from build123d import *

# Parameters (mm, degrees)
SKETCH_1_W             = 248
SKETCH_1_H             = 80
SM_BASE_FLANGE_1_DEPTH = 3
SKETCH_6_R             = 2
CUT_EXTRUDE_1_DEPTH    = 10
OTHER_START            = -40
OTHER_1_DEPTH          = 80
OTHER_1_2_DEPTH        = 80
CUT_EXTRUDE_2_DEPTH    = 10
FILLET_1_R             = 5


# Read off the part's stored shape, not the designer's step: 绘制的折弯1
# Sheet-metal steps are written as plain solids
with BuildPart() as part:
    # Sketch 1 → 基体-法兰1 (new body)
    with BuildSketch(Plane.XY):
        Rectangle(SKETCH_1_W, SKETCH_1_H)
    extrude(amount=-SM_BASE_FLANGE_1_DEPTH)

    # 草图6 → 切除-拉伸1 (cut)
    with BuildSketch(Plane.XY):
        with Locations((-97, 32)):
            Circle(SKETCH_6_R)
        with Locations((-76, 31)):
            Circle(SKETCH_6_R)
        with Locations((97, 32)):
            Circle(SKETCH_6_R)
        with Locations((76, 31)):
            Circle(SKETCH_6_R)
        with Locations((76, -31)):
            Circle(SKETCH_6_R)
        with Locations((97, -32)):
            Circle(SKETCH_6_R)
        with Locations((-97, -32)):
            Circle(SKETCH_6_R)
        with Locations((-76, -31)):
            Circle(SKETCH_6_R)
    extrude(amount=-CUT_EXTRUDE_1_DEPTH, mode=Mode.SUBTRACT)

    # Other 1 outline → Other 1 (cut)
    with BuildSketch(Plane(origin=(0, 0, 0), x_dir=(1, 0, 0), z_dir=(0, 1, 0)).offset(OTHER_START)):
        with BuildLine():
            Line((124, 3), (109, 3))
            ThreePointArc((109, 3), (112, 2.196152423), (114.196152423, 0))
            Line((114.196152423, 0), (124, 0))
            Line((124, 0), (124, 3))
        make_face()
        with BuildLine():
            ThreePointArc((-114.196152423, 0), (-112, 2.196152423), (-109, 3))
            Line((-109, 3), (-124, 3))
            Line((-124, 3), (-124, 0))
            Line((-124, 0), (-114.196152423, 0))
        make_face()
    extrude(amount=OTHER_1_DEPTH, mode=Mode.SUBTRACT)

    # Other 1 2 outline → Other 1 2 (add)
    with BuildSketch(Plane(origin=(0, 0, 0), x_dir=(1, 0, 0), z_dir=(0, 1, 0)).offset(OTHER_START)):
        with BuildLine():
            ThreePointArc((115, -3), (114.795554958, -1.447085729), (114.196152423, 0))
            Line((114.196152423, 0), (109, 0))
            ThreePointArc((109, 0), (111.121320344, -0.878679656), (112, -3))
            Line((112, -3), (112, -10.931416529))
            Line((112, -10.931416529), (115, -10.931416529))
            Line((115, -10.931416529), (115, -3))
        make_face()
        with BuildLine():
            Line((-109, 0), (-114.196152423, 0))
            ThreePointArc((-114.196152423, 0), (-114.795554958, -1.447085729), (-115, -3))
            Line((-115, -3), (-115, -10.931416529))
            Line((-115, -10.931416529), (-112, -10.931416529))
            Line((-112, -10.931416529), (-112, -3))
            ThreePointArc((-112, -3), (-111.121320344, -0.878679656), (-109, 0))
        make_face()
    extrude(amount=OTHER_1_2_DEPTH)

    # 草图8 → 切除-拉伸2 (cut)
    with BuildSketch(Plane(origin=(0, 0, -3), x_dir=(-1, 0, 0), z_dir=(0, 0, -1))):
        with BuildLine():
            Line((-52, 25), (52, 25))
            ThreePointArc((52, 25), (77, 0), (52, -25))
            Line((52, -25), (-52, -25))
            ThreePointArc((-52, -25), (-77, 0), (-52, 25))
        make_face()
    extrude(amount=-CUT_EXTRUDE_2_DEPTH, mode=Mode.SUBTRACT)

    # 圆角1
    fillet_1_edges = [part.edges().sort_by_distance(p)[0] for p in [
        (113.5, 40, 10.931416529),
        (113.5, -40, 10.931416529),
        (-113.5, -40, 10.931416529),
        (-113.5, 40, 10.931416529),
    ]]
    fillet(fillet_1_edges, radius=FILLET_1_R)


solid = part.part
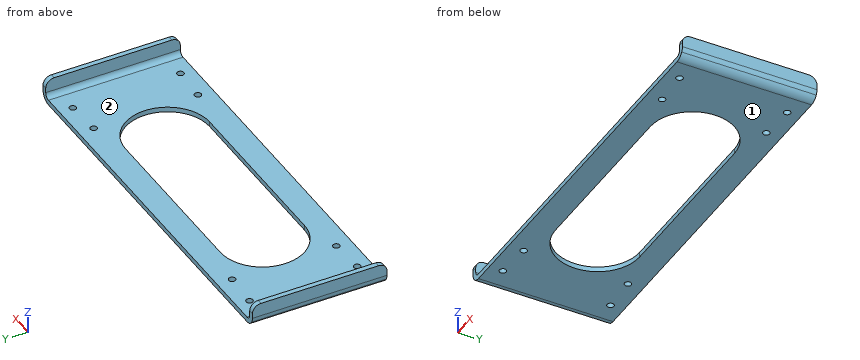
Could you check a few things on this model? Use its own coordinates, in mm. Face numbers are marked on the shaded views. Give positions to 0.01 mm unless a question says otherwise; leave off trailing zeros. Order: outer loops, then holes, each group sorted by start corner. A loop starts at its lowest first (then second) coordinate and runs counter-clockwise, first axis right, second up. Notation, with made-up numbers: (-1, 29) -> (27, 29) arc R26 cw to (27, 54) -> close; hole circle Ø2 at (65, 11.5). An arc over 180 degrees is marked (long way). Answer in a Markdown table with one row per item. Add a question column.
Item 1: Imagine slicing it at C-C (x = 97). List the corners of the cut face in (y, z) for me, and give its area (3 significant figures).
Item 2: Imagine slicing it at D-D (y = -19). List the corners of the cut face in (x, z) for me.
Item 3: We'd pull the mould along X, two halves only. Please class the marked faces 1 and 2: pulls with the +X half, pulls with the -X half, needs draft (parallel to the pull), parting line crosses it, or undercut.
Item 4: Imagine slicing it at A-A (y = 0). List the corners of the cut face in (x, z) for me.
Item 5: Imagine slicing it at B-B (x = 12.5). List the corners of the cut face in (y, z) for me, and give its area (3 significant figures).
Item 6: Please list where these lines run through material, in increasing order: probe 1 along Y at (x, z) = (97, -0.8); probe 2 along X at (y, z) = (3, 9); probe 3 along Y at (x, z) = (48, -1).
Item 7: I'm going to push a flat-ended pin straight in: P1, Ø4.5, axis at x = 76, y = -31, coming from the +Z side. Where does the tip first touch, or does it pass through?
Result:
| question | item | result |
|---|---|---|
| 1 | outline | (-40, -3) -> (-34, -3) -> (-34, 0) -> (-40, 0) -> close; (-30, -3) -> (30, -3) -> (30, 0) -> (-30, 0) -> close; (34, -3) -> (40, -3) -> (40, 0) -> (34, 0) -> close |
| 1 | area | 216 mm2 |
| 2 | outline | (-115, 3) arc R6 ccw to (-109, -3) -> (-68.25, -3) -> (-68.25, 0) -> (-109, 0) arc R3 cw to (-112, 3) -> (-112, 10.93) -> (-115, 10.93) -> close; (68.25, -3) -> (109, -3) arc R6 ccw to (115, 3) -> (115, 10.93) -> (112, 10.93) -> (112, 3) arc R3 cw to (109, 0) -> (68.25, 0) -> close |
| 3 | face 1 | needs draft |
| 3 | face 2 | undercut |
| 4 | outline | (-115, 3) arc R6 ccw to (-109, -3) -> (-77, -3) -> (-77, 0) -> (-109, 0) arc R3 cw to (-112, 3) -> (-112, 10.93) -> (-115, 10.93) -> close; (77, -3) -> (109, -3) arc R6 ccw to (115, 3) -> (115, 10.93) -> (112, 10.93) -> (112, 3) arc R3 cw to (109, 0) -> (77, 0) -> close |
| 5 | outline | (-40, -3) -> (-25, -3) -> (-25, 0) -> (-40, 0) -> close; (25, -3) -> (40, -3) -> (40, 0) -> (25, 0) -> close |
| 5 | area | 90.0 mm2 |
| 6 | probe 1 | -40 to -34, -30 to 30, 34 to 40 |
| 6 | probe 2 | -115 to -112, 112 to 115 |
| 6 | probe 3 | -40 to -25, 25 to 40 |
| 7 | P1 | z = 0 |
